```python
from build123d import *

# Parameters (mm, degrees)
SCHIZZO1_R                   = 1.725
ESTRUSIONE_ESTRUSIONE1_DEPTH = 3.8
SCHIZZO2_R                   = 1.725
ESTRUSIONE_ESTRUSIONE2_DEPTH = 7.5
SCHIZZO4_R                   = 3.1
TAGLIO_ESTRUSIONE1_DEPTH     = 5.65
SCHIZZO5_R                   = 5
ESTRUSIONE_ESTRUSIONE3_DEPTH = 0.5
SCHIZZO6_R                   = 3.9
ESTRUSIONE_ESTRUSIONE4_DEPTH = 7
SCHIZZO7_R                   = 2.2
TAGLIO_ESTRUSIONE2_DEPTH     = 25.75240203
TAGLIO_ESTRUSIONE3_DEPTH     = 25.75240203
TAGLIO_ESTRUSIONE4_DEPTH     = 27.938599166


with BuildPart() as part:
    # Schizzo1 → Estrusione-Estrusione1 (new body)
    with BuildSketch(Plane.XY):
        Polygon((-21.15, 1.7675), (-16.78, 6.1375), (21.15, 6.1375), (21.15, -6.1375), (-21.15, -6.1375), align=None)
        with Locations(Location((-15.5, 0.4875, 0), (0, 0, 180))):
            Circle(SCHIZZO1_R, mode=Mode.SUBTRACT)
    extrude(amount=ESTRUSIONE_ESTRUSIONE1_DEPTH)

    # Schizzo2 → Estrusione-Estrusione2 (add)
    # profile 1 of 2: a face of its own
    with BuildSketch(Plane.XY.offset(3.8)):
        with BuildLine():
            Line((-10.016361615, 6.1375), (-16.78, 6.1375))
            Line((-16.78, 6.1375), (-21.15, 1.7675))
            Line((-21.15, 1.7675), (-21.15, -6.1375))
            Line((-21.15, -6.1375), (-9.399966755, -6.1375))
            ThreePointArc((-9.399966755, -6.1375), (-11.485528203, -0.089251164), (-10.016361615, 6.1375))
        make_face()
        with Locations(Location((-15.5, 0.4875, 0), (0, 0, 180))):
            Circle(SCHIZZO2_R, mode=Mode.SUBTRACT)
    # profile 2 of 2: a face of its own
    with BuildSketch(Plane.XY.offset(3.8)):
        with BuildLine():
            Line((9.399966755, -6.1375), (21.15, -6.1375))
            Line((21.15, -6.1375), (21.15, 6.1375))
            Line((21.15, 6.1375), (10.016361615, 6.1375))
            ThreePointArc((10.016361615, 6.1375), (11.485528203, -0.089251164), (9.399966755, -6.1375))
        make_face()
    extrude(amount=ESTRUSIONE_ESTRUSIONE2_DEPTH)

    # Schizzo4 → Taglio-Estrusione1 (cut)
    with BuildSketch(Plane.XY.offset(11.3)):
        with Locations((-15.5, 0.4875)):
            Circle(SCHIZZO4_R)
    extrude(amount=-TAGLIO_ESTRUSIONE1_DEPTH, mode=Mode.SUBTRACT)

    # Schizzo5 → Estrusione-Estrusione3 (add)
    with BuildSketch(Plane.XY.offset(3.8)):
        with Locations(Location((0, 0.4875, 0), (0, 0, 180))):
            Circle(SCHIZZO5_R)
    extrude(amount=ESTRUSIONE_ESTRUSIONE3_DEPTH)

    # Schizzo6 → Estrusione-Estrusione4 (add)
    with BuildSketch(Plane.XY.offset(4.3)):
        with Locations((0, 0.4875)):
            Circle(SCHIZZO6_R)
    extrude(amount=ESTRUSIONE_ESTRUSIONE4_DEPTH)

    # Schizzo7 → Taglio-Estrusione2 (cut, through all)
    with BuildSketch(Plane.XY.offset(11.3)):
        with Locations((0, 0.4875)):
            Circle(SCHIZZO7_R)
    extrude(amount=-TAGLIO_ESTRUSIONE2_DEPTH, mode=Mode.SUBTRACT)

    # Schizzo8 → Taglio-Estrusione3 (cut, through all)
    with BuildSketch(Plane.XY.offset(11.3)):
        with BuildLine():
            Line((21.15, -6.1375), (21.15, -1.1616))
            ThreePointArc((21.15, -1.1616), (12.330643665, -2.247470782), (4.341411274, -6.1375))
            Line((4.341411274, -6.1375), (21.15, -6.1375))
        make_face()
    extrude(amount=-TAGLIO_ESTRUSIONE3_DEPTH, mode=Mode.SUBTRACT)

    # Schizzo9 → Taglio-Estrusione4 (cut, through all)
    with BuildSketch(Plane(origin=(0, 6.1375, 0), x_dir=(1, 0, 0), z_dir=(0, 1, 0))):
        with BuildLine():
            Line((17.15, -7.59), (15.15, -7.59))
            ThreePointArc((15.15, -7.59), (13.45, -5.89), (15.15, -4.19))
            Line((15.15, -4.19), (17.15, -4.19))
            ThreePointArc((17.15, -4.19), (18.85, -5.89), (17.15, -7.59))
        make_face()
    extrude(amount=-TAGLIO_ESTRUSIONE4_DEPTH, mode=Mode.SUBTRACT)


solid = part.part
```
Part model, mm, in its own coordinate system. A direction names the side the tool comes from. Round coordinates to 2 decimals unless told otherwise and drop trailing zeros. Write each loop counter-clockwise with the first axis right and the second up, starting at its lowest first coordinate (ties: lowest second). Pieces come first, ordered by that corner, then holes. Notation, with made-up numbers: (84.25, 71) -> (108.25, 71) arc R25 ccw to (108.25, 109) -> close; hole circle Ø2 at (88.5, 68). An arc over 180 degrees is marked (long way). Return JSON: item names as keys, results as strings. Group by question number.
Q1. Saw through at D-D on x = -15.5. Write the cut outline in (y, z), plus the area to 3 significant figures.
Q2. Mould opens along Y. For faces 1 (the flat face through (21.15, 3, 6)), 2 (the flat face through (-14, -1, 5.65)), 3 (the flat face through (-18.934, 3.983, 5.571)) say: pulls with the +Y half, pulls with the -Y half, needs draft (parallel to the pull), parting line crosses it, or undercut.
Q3. Saw through at B-B on y = -0.75. State how many separate pieces and enclosed holes the cut face has, plus the area to 3 significant figures.
Q4. Probe L1, parallel to Y at x = 0, z = 8.5; L2, parallel to Y at x = -15.5, z = 3.65; L3, parallel to X at y = 1, z = 5.25. List the from-to ranges inside material, lowest first. Write a range as [from, to].
Q5. Which spindle directions (+Z, -Z, +X, -X, +Y, -Y) get a long thin tool onto all of the face, cutting with end or side? Do faces 4 (the cylindrical face through (-13.777, 0.412, 2.785)), 5 (the cylindrical face through (11.41, 1.91, 7.5)), 6 (the flat face through (16, 2, 4.19)). Say none if no direction does.
Q6. Pin check, flat tips, straight feed: pin 1 (2 mm diameter, centred on y = 4.5, z = 6, fed in from -X); pin 2 (1.9 mm diameter, centred on x = -16.5, y = -0.5, fed in from +Z); pin 3 (4 mm diameter, centred on x = 0, y = 0.49, fed in from +Z). Stop position of each tip, or through.
Q7. Saw through at A-A on x = 0. Write the cut outline in (y, z), plus the area to 3 significant figures.
Answer:
{
 "1": {"outline": "(-6.14, 0) -> (-1.24, 0) -> (-1.24, 5.65) -> (-2.61, 5.65) -> (-2.61, 11.3) -> (-6.14, 11.3) -> close; (2.21, 0) -> (6.14, 0) -> (6.14, 11.3) -> (3.59, 11.3) -> (3.59, 5.65) -> (2.21, 5.65) -> close", "area": "84.2 mm2"},
 "2": {"face 1": "needs draft", "face 2": "undercut", "face 3": "pulls with the +Y half"},
 "3": {"separate pieces": "3", "enclosed holes": "1", "area": "260 mm2"},
 "4": {"L1": "[-3.41, -1.71], [2.69, 4.39]", "L2": "[-6.14, -1.24], [2.21, 6.14]", "L3": "[-21.15, -17.15], [-13.85, -11.49], [-3.87, -2.14], [2.14, 3.87], [11.49, 13.58], [18.72, 21.15]"},
 "5": {"face 4": "+Z, -Z", "face 5": "+Z", "face 6": "+Y, -Y"},
 "6": {"pin 1": "x = -19.42", "pin 2": "z = 5.65", "pin 3": "through"},
 "7": {"outline": "(-6.14, 0) -> (-1.71, 0) -> (-1.71, 11.3) -> (-3.41, 11.3) -> (-3.41, 4.3) -> (-4.51, 4.3) -> (-4.51, 3.8) -> (-6.14, 3.8) -> close; (2.69, 0) -> (6.14, 0) -> (6.14, 3.8) -> (5.49, 3.8) -> (5.49, 4.3) -> (4.39, 4.3) -> (4.39, 11.3) -> (2.69, 11.3) -> close", "area": "56.5 mm2"}
}
